Read the model definition and answer for the solid it produces. Units are mm, in the model's axes. A direction names the side the tool comes from. Coordinates: 2 decimals unless noted, no trailing zeros. Write each loop counter-clockwise with the first axis right and the second up, starting at its lowest first coordinate (ties: lowest second). Pieces come first, ordered by that corner, then holes.
(1) The part is cut by section C-C, the plane y = 10. Determine the outline of the cut face in (x, z), and give its area (3 significant figures).
(2) The part is cut by section B-B, the plane y = 5.25. Determine the outline of the cut face in (x, z), and give its area (4 significant figures).
(3) Which of the six approach directions +Z, -Z, +X, -X, +Y, -Y give full straight-line access (tool end or side, diameter ignored) to faces 4 (the flat face through (0, -2, -27.2)), 5 (the cylindrical face through (-5.361, 14.245, -7.969)), 6 (the flat face through (0, 0, -21)), 7 (the flat face through (0, 6, -9.3)), 8 (the flat face through (-7.5, 0, -8))?
(4) The part is cut by section D-D, the plane z = 3.5. Determine the outline of the cut face in (x, y).
(5) Given pin 1 (4 mm diameter, centred on x = -3.5, z = -14, fed in from +Y); pin 2 (1.9 mm diameter, centred on x = -1, z = -11.5, fed in from +Y); pin 3 (4.5 mm diameter, centred on x = 0.5, y = 6, fed in from +Z); pin 4 (5 mm diameter, centred on x = -1.5, z = -3.5, fed in from +Y), each flat-ended and moving along its own axis, determine where each tip first touches the part or whether it passes through.
(6) Straight lines are drawn through the part: line 1 along Z through (x, y) = (2.5, 6); line 2 along Z through (x, y) = (-4, -2.75); line 3 along Y through (x, z) = (0, -0.55). For each, find the intervals that lie inside material, in ascending order.
(7) Determine the mould class of faces 1 (the flat face through (-5, -2, -26)), 2 (the flat face through (0, 7, 0)), 3 (the cylindrical face through (5.245, 14.361, -7.969)) for opening direction Z: pulls with the +Z half, pulls with the -Z half, needs draft (parallel to the pull), parting line crosses it, or undercut.
(8) The part is cut by section A-A, the plane y = -0.75. Determine the outline of the cut face in (x, z).
Autodesk Inventor part; units mm, degrees
ref_plane "YZ Plane" through (0, 0, 0) normal (1, 0, 0) x (0, 1, 0)
ref_plane "XZ Plane" through (0, 0, 0) normal (0, 1, 0) x (-1, 0, 0)
ref_plane "XY Plane" through (0, 0, 0) normal (0, 0, 1) x (1, 0, 0)
sketch "Sketch4" plane through (0, 0, 0) normal (0, 0, 1) x (1, 0, 0)
  line L0 (-10.5, 0) -> (10.5, 0)
  line L1 (0, -3.3) -> (0, 19.8)
  line L2 (-7.5, 0) -> (7.5, 0)
  line L3 (7.5, 0) -> (7.5, 16.5)
  line L4 (7.5, 16.5) -> (-7.5, 16.5)
  line L5 (-7.5, 16.5) -> (-7.5, 0)
  circle A0 centre (0, 10) radius 2.5
  point P0 (0, 0)
  dimension "d0" = 7.5
  dimension "d1" = 7.5
  dimension "d2" = 16.5
  dimension "d3" = 5
  dimension "d4" = 6.5
extrude "Extrusion1" add sketch "Sketch4" against normal blind 15.9 contours L5 L4 L1 A0 L0 | L1 A0 L4 L3 L0
fillet "Fillet1" radius 7.5 2 edges at (7.5, 16.5, -7.95) (-7.5, 16.5, -7.95)
sketch "Sketch10" plane through (-7.5, 0, 0) normal (0, -1, 0) x (1, 0, 0)
  line L0 (-3, 0) -> (18, 0)
  line L1 (7.5, -19.08) -> (7.5, 3.18)
  line L2 (15, 12.05) -> (0, 12.05)
  line L3 (0, 12.05) -> (0, -27.95)
  line L4 (0, -27.95) -> (15, -27.95)
  line L5 (15, -27.95) -> (15, 12.05)
  line L6 (11.5, 11.05) -> (3.5, 11.05)
  line L7 (2.5, 10.05) -> (2.5, 9.05)
  line L8 (3.5, 8.05) -> (11.5, 8.05)
  line L9 (12.5, 9.05) -> (12.5, 10.05)
  line L10 (15, 0) -> (15, -15.9)
  line L11 (15, -8.075) -> (0, -8.075)
  line L12 (0, -15.9) -> (0, 0)
  line L13 (11.5, -27.2) -> (3.5, -27.2)
  line L14 (2.5, -26.2) -> (2.5, -25.2)
  line L15 (3.5, -24.2) -> (11.5, -24.2)
  line L16 (12.5, -25.2) -> (12.5, -26.2)
  arc A0 (11.5, 8.05) -> (12.5, 9.05) centre (11.5, 9.05) ccw
  arc A1 (12.5, 10.05) -> (11.5, 11.05) centre (11.5, 10.05) ccw
  arc A2 (3.5, 11.05) -> (2.5, 10.05) centre (3.5, 10.05) ccw
  arc A3 (2.5, 9.05) -> (3.5, 8.05) centre (3.5, 9.05) ccw
  arc A4 (12.5, -25.2) -> (11.5, -24.2) centre (11.5, -25.2) ccw
  arc A5 (11.5, -27.2) -> (12.5, -26.2) centre (11.5, -26.2) ccw
  arc A6 (3.5, -24.2) -> (2.5, -25.2) centre (3.5, -25.2) ccw
  arc A7 (2.5, -26.2) -> (3.5, -27.2) centre (3.5, -26.2) ccw
  point P0 (7.5, 0)
  point P1 (12.5, 11.05)
  point P2 (2.5, 8.05)
  point P3 (2.5, 11.05)
  point P4 (12.5, 8.05)
  point P5 (15, -6.55)
  point P6 (15, -9.6)
  point P7 (0, -9.6)
  point P8 (0, -6.55)
  point P9 (12.5, -27.2)
  point P10 (2.5, -24.2)
  point P11 (2.5, -27.2)
  point P12 (12.5, -24.2)
  point P13 (15, -2.8)
  dimension "d20" = 15
  dimension "d21" = 40
  dimension "d22" = 12.05
  dimension "d23" = 7.5
  dimension "d24" = 3
  dimension "d25" = 1
  dimension "d26" = 10
  dimension "d27" = 2.5
  dimension "d28" = 8.075
  dimension "d29" = 1
extrude "Extrusion5" add sketch "Sketch10" along normal blind 4
sketch "Sketch13" plane through (7.5, 9, 0) normal (1, 0, 0) x (0, 0, -1)
  line L0 (0, -17.1) -> (0, 11.6)
  line L1 (35.95, -9) -> (-20.05, -9)
  line L2 (0, -9) -> (0, 0)
  line L3 (0, 7.5) -> (15.9, 7.5)
  line L4 (0, -9) -> (2.7, -9)
  line L5 (2.7, -9) -> (2.7, 7.5)
  line L6 (2.7, 7.5) -> (0, 7.5)
  line L7 (0, 7.5) -> (0, -9)
  line L8 (15.9, -9) -> (15.9, 0)
  line L9 (15.9, -9) -> (13.2, -9)
  line L10 (13.2, -9) -> (13.2, 7.5)
  line L11 (13.2, 7.5) -> (15.9, 7.5)
  line L12 (15.9, 7.5) -> (15.9, -9)
  line L13 (6.6, -9) -> (9.3, -9)
  line L14 (9.3, -9) -> (9.3, 7.5)
  line L15 (9.3, 7.5) -> (6.6, 7.5)
  line L16 (6.6, 7.5) -> (6.6, -9)
  dimension "d47" = 2.7
  dimension "d48" = 2.7
  dimension "d49" = 2.7
  dimension "d50" = 15.9
  dimension "d51" = 3.9
  dimension "d52" = 3.9
extrude "Extrusion8" cut sketch "Sketch13" against normal through all contours L5 L3 L16 L1 | L14 L3 L10 L1
properties part number "droneMount"
Computed:
1. outline: (-7.43, -15.9) - (-2.5, -15.9) - (-2.5, -13.2) - (-7.43, -13.2) - close; (-7.43, -9.3) - (-2.5, -9.3) - (-2.5, -6.6) - (-7.43, -6.6) - close; (-7.43, -2.7) - (-2.5, -2.7) - (-2.5, 0) - (-7.43, 0) - close; (2.5, -15.9) - (7.43, -15.9) - (7.43, -13.2) - (2.5, -13.2) - close; (2.5, -9.3) - (7.43, -9.3) - (7.43, -6.6) - (2.5, -6.6) - close; (2.5, -2.7) - (7.43, -2.7) - (7.43, 0) - (2.5, 0) - close
1. area: 79.9 mm2
2. outline: (-7.5, -15.9) - (7.5, -15.9) - (7.5, -13.2) - (-7.5, -13.2) - close; (-7.5, -9.3) - (7.5, -9.3) - (7.5, -6.6) - (-7.5, -6.6) - close; (-7.5, -2.7) - (7.5, -2.7) - (7.5, 0) - (-7.5, 0) - close
2. area: 121.5 mm2
3. face 4: +Y, -Y
3. face 5: +Z, -Z, -X, +Y
3. face 6: -Z, +X, -X, +Y
3. face 7: +X, -X, +Y
3. face 8: +Z, -Z, -X, +Y, -Y
4. outline: (-7.5, -4) - (7.5, -4) - (7.5, 0) - (-7.5, 0) - close
5. pin 1: stops at y = 16.35
5. pin 2: stops at y = 0
5. pin 3: stops at z = 0
5. pin 4: stops at y = 16.5
6. line 1: z = -15.9 to -13.2, -9.3 to -6.6, -2.7 to 0
6. line 2: z = -27.95 to -27.2, -24.2 to 8.05, 11.05 to 12.05
6. line 3: y = -4 to 7.5, 12.5 to 16.5
7. face 1: undercut
7. face 2: pulls with the +Z half
7. face 3: needs draft
8. outline: (-7.5, -27.95) - (7.5, -27.95) - (7.5, 12.05) - (-7.5, 12.05) - close; hole (-5, -26.2) arc R1 ccw to (-4, -27.2) - (4, -27.2) arc R1 ccw to (5, -26.2) - (5, -25.2) arc R1 ccw to (4, -24.2) - (-4, -24.2) arc R1 ccw to (-5, -25.2) - close; hole (-5, 9.05) arc R1 ccw to (-4, 8.05) - (4, 8.05) arc R1 ccw to (5, 9.05) - (5, 10.05) arc R1 ccw to (4, 11.05) - (-4, 11.05) arc R1 ccw to (-5, 10.05) - close
